Design review of the part built by this model. Coordinates are the model's own, in mm. Face numbers are marked on the shaded views. A direction names the side the tool comes from. Coordinates: 2 decimals unless noted, no trailing zeros. Order: outer loops, then holes, each group sorted by start corner. A loop starts at its lowest first (then second) coordinate and runs counter-clockwise, first axis right, second up. Notation, with made-up numbers: (-13.75, 12.25) -> (6.25, 12.25) arc R30 ccw to (6.25, 42.25) -> close; hole circle Ø10 at (-13, 75.25). An arc over 180 degrees is marked (long way). Use a Markdown table: item, result. Add a question column.
Q1. Add section D-D (z = -7). State the section outline as (x, y) points, then the cut area to 3 significant figures.
Q2. Add section A-A (z = 0). State the section outline as (x, y) points (3 decimals).
Q3. Insertion check: pin 1 (1.6 mm diameter, centred on x = -17.5, z = 17.5, fed in from -Y); pin 2 (1.6 mm diameter, centred on y = 3, z = 17.5, fed in from +X); pin 3 (2.5 mm diameter, centred on x = 5, y = 3.5, fed in from +Z); pin 4 (1.5 mm diameter, centred on x = -5.5, z = -8, fed in from +Y). Each pin has a flat end and moves straight along its axis. Give the tip position at first contact, or say it passes through.
Q4. Wall thickness on probe 1 along X at (y, z) = (0.55, 0) (3 decimals); probe 2 along Y at (x, z) = (-3.5, 2); probe 3 along Z at (x, y) = (-21, 4.8): over which ranges is each line inside the solid? List them lowest first.
Q5. Machinability: for the marked faces 1 and 2, which of the approach directions +Z, -Z, +X, -X, +Y, -Y give a long, thin tool a straight path to every point of the face, cutting with its end or side? Answer none if there is none.
Q6. Add section B-B (y = 3.1). State the section outline as (x, z) points.
Q7. Add section C-C (x = 2). State the section outline as (y, z) points.
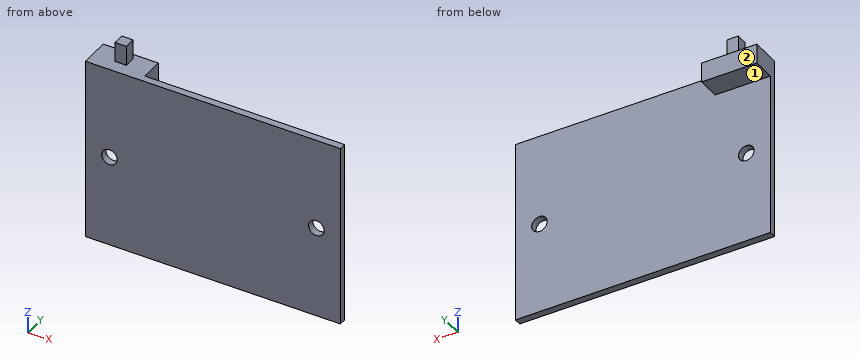
from build123d import *

# Parameters (mm, degrees)
SKETCH1_W           = 45.72
SKETCH1_H           = 33.02
SKETCH1_R           = 1.397
BOSS_EXTRUDE1_DEPTH = 1.27
SKETCH3_W           = 9.906
SKETCH3_H           = 3.556
BOSS_EXTRUDE2_DEPTH = 4.064
SKETCH4_W           = 2.032
SKETCH4_H           = 2.032
BOSS_EXTRUDE3_DEPTH = 3.556


with BuildPart() as part:
    # Sketch1 → Boss-Extrude1 (new body)
    with BuildSketch(Plane(origin=(0, 0, 0), x_dir=(1, 0, 0), z_dir=(0, 1, 0))):
        Rectangle(SKETCH1_W, SKETCH1_H)
        with Locations(Location((-18.542, 0, 0), (0, 0, 270))):
            Circle(SKETCH1_R, mode=Mode.SUBTRACT)
        with Locations(Location((18.542, 0, 0), (0, 0, 270))):
            Circle(SKETCH1_R, mode=Mode.SUBTRACT)
    extrude(amount=BOSS_EXTRUDE1_DEPTH)

    # Sketch3 → Boss-Extrude2 (add)
    with BuildSketch(Plane(origin=(0, 1.27, 0), x_dir=(1, 0, 0), z_dir=(0, 1, 0))):
        with Locations((-17.907, -14.732)):
            Rectangle(SKETCH3_W, SKETCH3_H)
    extrude(amount=BOSS_EXTRUDE2_DEPTH)

    # Sketch4 → Boss-Extrude3 (add)
    with BuildSketch(Plane.XY.offset(16.51)):
        with Locations((-17.907, 3.302)):
            Rectangle(SKETCH4_W, SKETCH4_H)
    extrude(amount=BOSS_EXTRUDE3_DEPTH)


solid = part.part
Established:
| question | item | result |
|---|---|---|
| 1 | outline | (-22.86, 0) -> (22.86, 0) -> (22.86, 1.27) -> (-22.86, 1.27) -> close |
| 1 | area | 58.1 mm^2 |
| 2 | outline | (-22.86, 0) -> (-19.939, 0) -> (-19.939, 1.27) -> (-22.86, 1.27) -> close; (-17.145, 0) -> (17.145, 0) -> (17.145, 1.27) -> (-17.145, 1.27) -> close; (19.939, 0) -> (22.86, 0) -> (22.86, 1.27) -> (19.939, 1.27) -> close |
| 3 | pin 1 | y = 2.29 |
| 3 | pin 2 | x = -16.89 |
| 3 | pin 3 | through |
| 3 | pin 4 | y = 1.27 |
| 4 | probe 1 | -22.86 to -19.939, -17.145 to 17.145, 19.939 to 22.86 |
| 4 | probe 2 | 0 to 1.27 |
| 4 | probe 3 | 12.95 to 16.51 |
| 5 | face 1 | -Z, +X, -X, +Y |
| 5 | face 2 | +Z, -Z, +X, -X, +Y |
| 6 | outline | (-22.86, 12.95) -> (-12.95, 12.95) -> (-12.95, 16.51) -> (-16.89, 16.51) -> (-16.89, 20.07) -> (-18.92, 20.07) -> (-18.92, 16.51) -> (-22.86, 16.51) -> close |
| 7 | outline | (0, -16.51) -> (1.27, -16.51) -> (1.27, 16.51) -> (0, 16.51) -> close |
